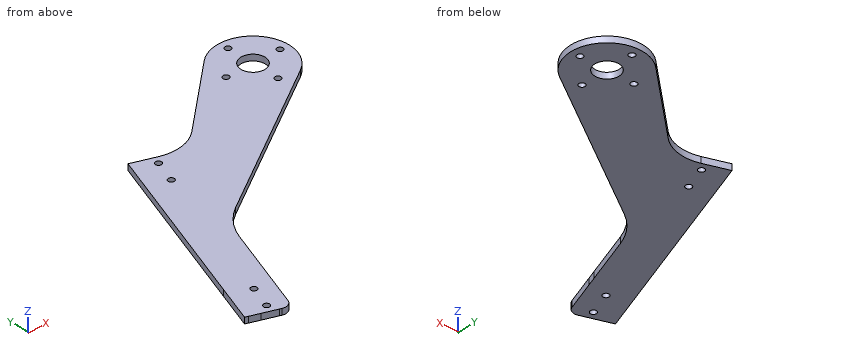
from build123d import *

# Parameters (mm, degrees)
MODEL_R         = 1.5
MODEL_R_2       = 6
EXTRUDE_1_DEPTH = 3


with BuildPart() as part:
    # Model → 凸台-拉伸1 (new body)
    with BuildSketch(Plane.XY):
        with BuildLine():
            Line((2489.401518441, 1758.026761836), (2477.832923788, 1762.20884815))
            Line((2477.832923788, 1762.20884815), (2447.235551014, 1677.569609145))
            Line((2447.235551014, 1677.569609145), (2443.835842928, 1668.165249256))
            Line((2443.835842928, 1668.165249256), (2440.436134842, 1658.760889367))
            Line((2440.436134842, 1658.760889367), (2441.846788825, 1658.250933154))
            Line((2441.846788825, 1658.250933154), (2446.54896877, 1656.551079111))
            Line((2446.54896877, 1656.551079111), (2453.602238687, 1654.001298046))
            Line((2453.602238687, 1654.001298046), (2454.542674676, 1653.661327237))
            ThreePointArc((2454.542674676, 1653.661327237), (2457.600929914, 1653.801533876), (2459.664301866, 1656.063187959))
            Line((2459.664301866, 1656.063187959), (2465.103834804, 1671.110163782))
            Line((2465.103834804, 1671.110163782), (2466.691626019, 1675.502352652))
            Line((2466.691626019, 1675.502352652), (2475.230094166, 1699.121682704))
            ThreePointArc((2475.230094166, 1699.121682704), (2480.022947289, 1707.670704716), (2487.315446875, 1714.218732526))
            Line((2487.315446875, 1714.218732526), (2566.313045726, 1764.584123777))
            ThreePointArc((2566.313045726, 1764.584123777), (2570.993188824, 1790.619216903), (2544.66757117, 1793.206042885))
            Line((2544.66757117, 1793.206042885), (2509.499643925, 1761.897465327))
            ThreePointArc((2509.499643925, 1761.897465327), (2499.983234073, 1757.196382583), (2489.401518441, 1758.026761836))
        make_face()
        with Locations((2451.67059596, 1658.952939832)):
            Circle(MODEL_R, mode=Mode.SUBTRACT)
        with Locations((2455.750245663, 1670.238171699)):
            Circle(MODEL_R, mode=Mode.SUBTRACT)
        with Locations((2482.267968734, 1743.592178837)):
            Circle(MODEL_R, mode=Mode.SUBTRACT)
        with Locations((2486.347618438, 1754.877410704)):
            Circle(MODEL_R, mode=Mode.SUBTRACT)
        with Locations((2556.636409551, 1766.261828225)):
            Circle(MODEL_R, mode=Mode.SUBTRACT)
        with Locations((2543.136409551, 1779.761828225)):
            Circle(MODEL_R, mode=Mode.SUBTRACT)
        with Locations((2556.636409551, 1779.761828225)):
            Circle(MODEL_R_2, mode=Mode.SUBTRACT)
        with Locations((2556.636409551, 1793.261828225)):
            Circle(MODEL_R, mode=Mode.SUBTRACT)
        with Locations((2570.136409551, 1779.761828225)):
            Circle(MODEL_R, mode=Mode.SUBTRACT)
    extrude(amount=EXTRUDE_1_DEPTH)


solid = part.part
Can you work these out from the model? Positions are in its coordinate system, mm. Round coordinates to 2 decimals unless told otherwise and drop trailing zeros. Loops run counter-clockwise (first coordinate to the right, second up) from the corner with the lowest first, then second, coordinate; pieces in that order, holes last. Notation, with made-up numbers: (78.25, 6) - (113.25, 6) arc R13 ccw to (113.25, 26) - close; hole circle Ø11 at (53, -5). An arc over 180 degrees is marked (long way). Answer in a Markdown table with one row per item. Add a question column.
Q1. I want a section at B-B on y = 1716.5. List the corners of the cut face in (x, z) for me.
Q2. For pin 1 Ø2.5 at (x, y) = (2482.27, 1743.59) entering from -Z; pin 2 Ø1.5 at (y, z) = (1724, 2) entering from -X, each with a flat end and sliding along its axis, tell me the tip position at first contact or that it passes through.
Q3. I need wall thicknesses on L1, parallel to Y at x = 2486.5, z = 0.45; L2, parallel to X at y = 1784.5, z = 0.55; L3, parallel to X at y = 1671.5, z = 2. Which ranges of each line are inside material? Lowest first, please.
Q4. I want a section at A-A on z = 1.7. Count the separate pieces of the cut face and the enclosed holes in it, and give its area (3 significant figures).
Q5. I want a section at C-C on x = 2500. List the corners of the cut face in (y, z) for me, and give its area (3 significant figures).
A:
| question | item | result |
|---|---|---|
| 1 | outline | (2461.31, 0) - (2490.89, 0) - (2490.89, 3) - (2461.31, 3) - close |
| 2 | pin 1 | through |
| 2 | pin 2 | x = 2463.75 |
| 3 | L1 | 1713.68 to 1753.39, 1756.37 to 1759.08 |
| 3 | L2 | 2534.89 to 2552.96, 2560.32 to 2574 |
| 3 | L3 | 2445.04 to 2454.94, 2456.56 to 2465.24 |
| 4 | separate pieces | 1 |
| 4 | enclosed holes | 9 |
| 4 | area | 5,070 mm^2 |
| 5 | outline | (1722.31, 0) - (1757.2, 0) - (1757.2, 3) - (1722.31, 3) - close |
| 5 | area | 105 mm^2 |
